Answer from the drawing. Dimensions are ordinates in mm from the lowest x, y and z of the part. A direction names the side the tool comes from. Coordinates: 2 decimals unless noted, no trailing zeros. Write each loop counter-clockwise with the first axis right and the second up, starting at its lowest first coordinate (ties: lowest second). Pieces come first, ordered by that corner, then holes. Notation, with made-up numbers: (-11.75, 59) -> (35.25, 59) arc R13 ccw to (35.25, 67) -> close; hole circle Ø2 at (-11, 88.25). An arc over 180 degrees is marked (long way). Answer as a JSON object with one key per item and string values. Group by question number.
(1) Find section A-A (y = 19). Give the vertices of the cut face in (x, z), then the cut area to 3 significant figures.
(2) Find section B-B (x = 15). Give the vertices of the cut face in (y, z) (1 decimal), then the cut area to 3 significant figures.
(3) For a pull along Z with two mould halves and no side action, classify the marked faces 1, 2, 3 and 4 as +Z half, -Z half, draft (parallel to the pull), parting line (faces both ways), or undercut.
(4) Straight lines are drawn through the part: L1, parallel to X at y = 22.5, z = 29; L2, parallel to Y at x = 26.25, z = 17.25; L3, parallel to Y at x = 13.25, z = 10.5. For each, find the intervals that lie inside material, in ascending order.
(5) Find section D-D (y = 11). Give the vertices of the cut face in (x, z).
(6) Which of the six approach directions +Z, -Z, +X, -X, +Y, -Y give full straight-line access (tool end or side, diameter ignored) to the marked faces 5 and 6?
(7) Find section C-C (z = 25.25). Give the vertices of the cut face in (x, y).
(8) Flat-ended cylindrical pins translate along their axes: P1, Ø13.5, axis at x = 12, z = 7, coming from the -Y side; P2, Ø1, axis at x = 18.5, y = 6, coming from the +Z side; P3, Ø10, axis at x = 15, z = 10.67, coming from the +Y side. Find the tip coordinate at first contact, or state that the pin passes through.
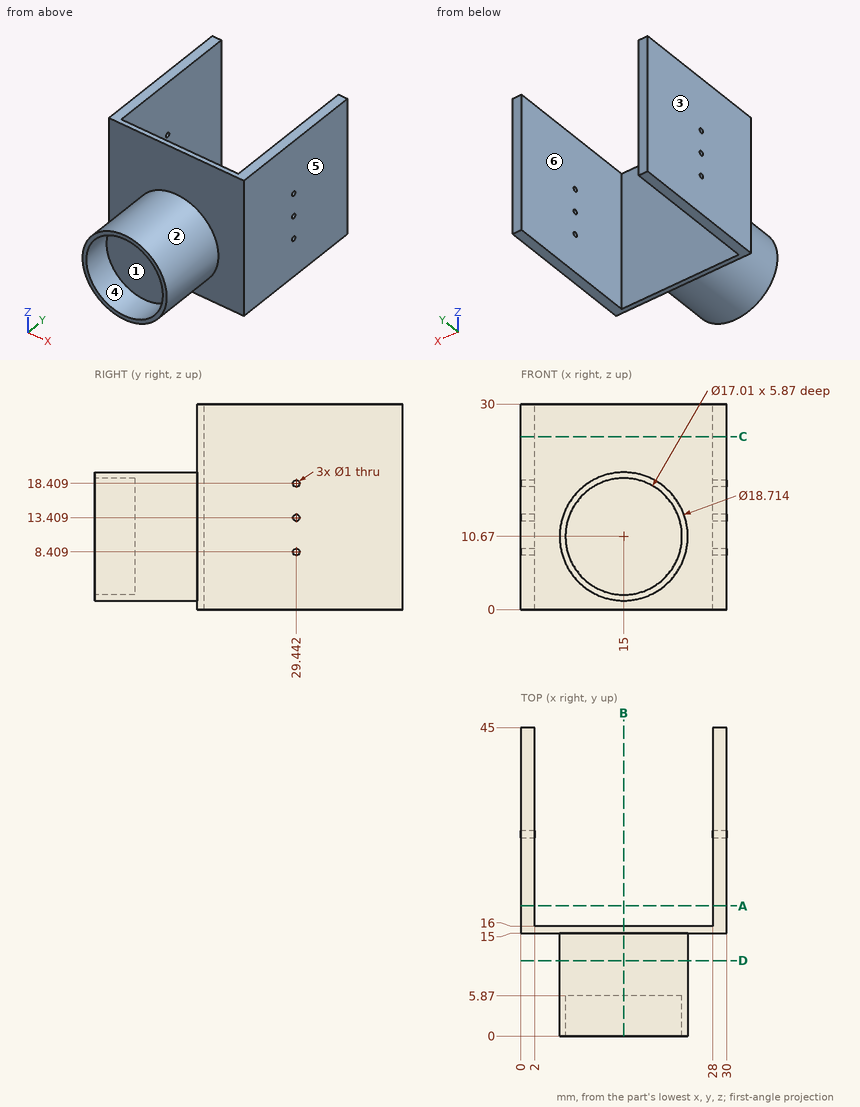
Results below:
{
 "1": {"outline": "(0, 0) -> (2, 0) -> (2, 30) -> (0, 30) -> close; (28, 0) -> (30, 0) -> (30, 30) -> (28, 30) -> close", "area": "120 mm2"},
 "2": {"outline": "(0, 1.3) -> (15, 1.3) -> (15, 0) -> (16, 0) -> (16, 30) -> (15, 30) -> (15, 20) -> (0, 20) -> (0, 19.2) -> (5.9, 19.2) -> (5.9, 2.2) -> (0, 2.2) -> close", "area": "211 mm2"},
 "3": {"face 1": "undercut", "face 2": "parting line", "face 3": "draft", "face 4": "undercut"},
 "4": {"L1": "x = 0 to 2, 28 to 30", "L2": "y = 15 to 16", "L3": "y = 5.87 to 16"},
 "5": {"outline": "circle Ø18.71 at (15, 10.67)"},
 "6": {"face 5": "+Z, -Z, +X, +Y, -Y", "face 6": "+Z, -Z, +Y"},
 "7": {"outline": "(0, 15) -> (30, 15) -> (30, 45) -> (28, 45) -> (28, 16) -> (2, 16) -> (2, 45) -> (0, 45) -> close"},
 "8": {"P1": "stops at y = 0", "P2": "stops at z = 19.53", "P3": "stops at y = 16"}
}
